```python
from build123d import *

# Parameters (mm, degrees)
SKETCH1_R           = 1.6
SKETCH1_W           = 21
SKETCH1_H           = 41
BOSS_EXTRUDE1_DEPTH = 11
SKETCH6_W           = 21
SKETCH6_H           = 0.1
CUT_EXTRUDE1_DEPTH  = 91.428148273
SKETCH7_W           = 21
SKETCH7_H           = 41.2
SKETCH7_R           = 1.6
CUT_EXTRUDE2_DEPTH  = 11
BOSS_EXTRUDE2_START = -11
SKETCH8_W           = 200
SKETCH8_H           = 250
SKETCH8_W_2         = 21
SKETCH8_H_2         = 41.2
SKETCH8_R           = 1.6
BOSS_EXTRUDE2_DEPTH = 11
FILLET1_R           = 64
FILLET2_R           = 64
FILLET3_R           = 64
FILLET4_R           = 64
SKETCH12_R          = 6.933523759
BOSS_EXTRUDE3_DEPTH = 19.05
SKETCH13_R          = 15
CUT_EXTRUDE3_DEPTH  = 11


with BuildPart() as part:
    # Sketch1 → Boss-Extrude1 (new body)
    with BuildSketch(Plane.XY):
        with BuildLine():
            Line((-20, 70), (-20, -50))
            ThreePointArc((-20, -50), (-2.5, -67.5), (15, -50))
            Line((15, -50), (15, 70))
            ThreePointArc((15, 70), (-2.5, 87.5), (-20, 70))
        make_face()
        with Locations((-7.5, 79.5)):
            Circle(SKETCH1_R, mode=Mode.SUBTRACT)
        with Locations(Location((2.5, 79.5, 0), (0, 0, 180))):
            Circle(SKETCH1_R, mode=Mode.SUBTRACT)
        with Locations((2.5, 30.5)):
            Circle(SKETCH1_R, mode=Mode.SUBTRACT)
        with Locations(Location((-7.5, 30.5, 0), (0, 0, 180))):
            Circle(SKETCH1_R, mode=Mode.SUBTRACT)
        with Locations((-2.5, 55)):
            Rectangle(SKETCH1_W, SKETCH1_H, mode=Mode.SUBTRACT)
    extrude(amount=BOSS_EXTRUDE1_DEPTH)

    # Sketch6 → Cut-Extrude1 (cut, through all)
    with BuildSketch(Plane.XY.offset(11)):
        with Locations((-2.5, 75.55)):
            Rectangle(SKETCH6_W, SKETCH6_H)
        with Locations((-2.5, 34.45)):
            Rectangle(SKETCH6_W, SKETCH6_H)
    extrude(amount=-CUT_EXTRUDE1_DEPTH, mode=Mode.SUBTRACT)

    # Sketch7 → Cut-Extrude2 (cut)
    with BuildSketch(Plane(origin=(0, 0, 0), x_dir=(-1, 0, 0), z_dir=(0, 0, -1))):
        with Locations((2.5, -35)):
            Rectangle(SKETCH7_W, SKETCH7_H)
        with Locations((-2.5, -10.5)):
            Circle(SKETCH7_R)
        with Locations((7.5, -10.5)):
            Circle(SKETCH7_R)
        with Locations((-2.5, -59.5)):
            Circle(SKETCH7_R)
        with Locations((7.5, -59.5)):
            Circle(SKETCH7_R)
    extrude(amount=-CUT_EXTRUDE2_DEPTH, mode=Mode.SUBTRACT)

    # Sketch8 → Boss-Extrude2 (add)
    # profile 1 of 6: a face of its own
    with BuildSketch(Plane.XY.offset(11).offset(BOSS_EXTRUDE2_START)):
        with Locations((-2.5, 55)):
            Rectangle(SKETCH8_W, SKETCH8_H)
        with BuildLine():
            ThreePointArc((-20, -50), (-2.5, -67.5), (15, -50))
            Line((15, -50), (15, 70))
            ThreePointArc((15, 70), (-2.5, 87.5), (-20, 70))
            Line((-20, 70), (-20, -50))
        make_face(mode=Mode.SUBTRACT)
    # profile 2 of 6: a face of its own
    with BuildSketch(Plane.XY.offset(11).offset(BOSS_EXTRUDE2_START)):
        with Locations((-2.5, -35)):
            Rectangle(SKETCH8_W_2, SKETCH8_H_2)
    # profile 3 of 6: a face of its own
    with BuildSketch(Plane.XY.offset(11).offset(BOSS_EXTRUDE2_START)):
        with Locations((-7.5, -59.5)):
            Circle(SKETCH8_R)
    # profile 4 of 6: a face of its own
    with BuildSketch(Plane.XY.offset(11).offset(BOSS_EXTRUDE2_START)):
        with Locations((2.5, -59.5)):
            Circle(SKETCH8_R)
    # profile 5 of 6: a face of its own
    with BuildSketch(Plane.XY.offset(11).offset(BOSS_EXTRUDE2_START)):
        with Locations((-7.5, -10.5)):
            Circle(SKETCH8_R)
    # profile 6 of 6: a face of its own
    with BuildSketch(Plane.XY.offset(11).offset(BOSS_EXTRUDE2_START)):
        with Locations((2.5, -10.5)):
            Circle(SKETCH8_R)
    extrude(amount=BOSS_EXTRUDE2_DEPTH)

    # Fillet1
    fillet1_edges = [part.edges().sort_by_distance(p)[0] for p in [
        (-102.5, 180, 5.5),
    ]]
    fillet(fillet1_edges, radius=FILLET1_R)

    # Fillet2
    fillet2_edges = [part.edges().sort_by_distance(p)[0] for p in [
        (97.5, 180, 5.5),
    ]]
    fillet(fillet2_edges, radius=FILLET2_R)

    # Fillet3
    fillet3_edges = [part.edges().sort_by_distance(p)[0] for p in [
        (97.5, -70, 5.5),
    ]]
    fillet(fillet3_edges, radius=FILLET3_R)

    # Fillet4
    fillet4_edges = [part.edges().sort_by_distance(p)[0] for p in [
        (-102.5, -70, 5.5),
    ]]
    fillet(fillet4_edges, radius=FILLET4_R)

    # Sketch12 → Boss-Extrude3 (add)
    with BuildSketch(Plane(origin=(0, 0, 0), x_dir=(-1, 0, 0), z_dir=(0, 0, -1))):
        with Locations(Location((67.5, 155, 0), (0, 0, 180))):
            Circle(SKETCH12_R)
        with Locations(Location((-62.5, -45, 0), (0, 0, 180))):
            Circle(SKETCH12_R)
        with Locations(Location((67.5, -45, 0), (0, 0, 180))):
            Circle(SKETCH12_R)
        with Locations(Location((-62.5, 155, 0), (0, 0, 180))):
            Circle(SKETCH12_R)
    extrude(amount=BOSS_EXTRUDE3_DEPTH)

    # Sketch13 → Cut-Extrude3 (cut)
    with BuildSketch(Plane.XY.offset(11)):
        with Locations((-62.5, 135)):
            Circle(SKETCH13_R)
        with Locations((57.5, 135)):
            Circle(SKETCH13_R)
        with Locations((57.5, -25)):
            Circle(SKETCH13_R)
        with Locations((-62.5, -25)):
            Circle(SKETCH13_R)
    extrude(amount=-CUT_EXTRUDE3_DEPTH, mode=Mode.SUBTRACT)


solid = part.part
```
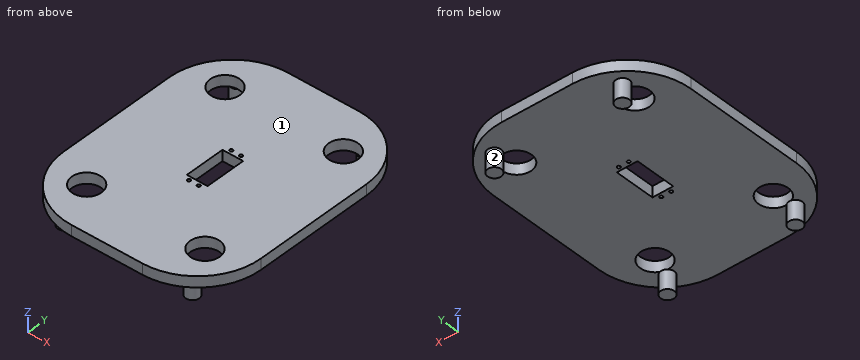
Part model, mm, in its own coordinate system. Face numbers are marked on the shaded views. Coordinates: 2 decimals unless noted, no trailing zeros. Order: outer loops, then holes, each group sorted by start corner. A loop starts at its lowest first (then second) coordinate and runs counter-clockwise, first axis right, second up. Notation, with made-up numbers: (-20, 77.5) - (10, 77.5) arc R8 cw to (10, 89.5) - close; hole circle Ø9 at (71.25, -10). An arc over 180 degrees is marked (long way). Return JSON: item names as keys, results as strings. Group by question number.
Item 1: Cut at B-B (z = -4). List the corners of the cut face in (x, y), plus the area to 3 significant figures.
Item 2: Cut at D-D (x = 19.5). List the corners of the cut face in (y, z).
Item 3: Pull direction X, two halves, no side cores. Call the marked faces 1 and 2: pulls with the +X half, pulls with the -X half, needs draft (parallel to the pull), parting line crosses it, or undercut.
Item 4: Cut at A-A (y = -15). List the corners of the cut face in (x, z), plus the area to 3 significant figures.
Item 5: Cut at C-C (y = 155). List the corners of the cut face in (x, z), plus the area to 3 significant figures.
Item 6: Pin check, flat tips, straight feed: pin 1 (4 mm diameter, centred on x = -7.5, y = 30.5, fed in from -Z); pin 2 (2 mm diameter, centred on x = -64.5, y = -38.5, fed in from +Z); pin 3 (5 mm diameter, centred on y = 153, z = 3.5, fed in from -X) (3 decimals). Stop position of each tip, or through.
Item 7: Drill centre lines: probe 1 along Y at (x, z) = (-7.5, 6.25); probe 2 along Y at (x, z) = (-5, 0.5); probe 3 along Y at (x, z) = (57, 7). Where is each one in solid material? Low to high. Write a range as from..to.
Check values:
{
 "1": {"outline": "circle Ø13.87 at (-67.5, -45); circle Ø13.87 at (-67.5, 155); circle Ø13.87 at (62.5, -45); circle Ø13.87 at (62.5, 155)", "area": "604 mm2"},
 "2": {"outline": "(-70, 0) - (180, 0) - (180, 11) - (-70, 11) - close"},
 "3": {"face 1": "needs draft", "face 2": "undercut"},
 "4": {"outline": "(-101.86, 0) - (-73.68, 0) - (-73.68, 11) - (-101.86, 11) - close; (-51.32, 0) - (46.32, 0) - (46.32, 11) - (-51.32, 11) - close; (68.68, 0) - (96.86, 0) - (96.86, 11) - (68.68, 11) - close", "area": "1,690 mm2"},
 "5": {"outline": "(-89.24, 0) - (-74.43, 0) - (-74.43, -19.05) - (-60.57, -19.05) - (-60.57, 0) - (55.57, 0) - (55.57, -19.05) - (69.43, -19.05) - (69.43, 0) - (84.24, 0) - (84.24, 11) - (-89.24, 11) - close", "area": "2,440 mm2"},
 "6": {"pin 1": "stops at z = 0", "pin 2": "stops at z = 0", "pin 3": "stops at x = -92.405"},
 "7": {"probe 1": "y = -70..28.9, 32.1..34.4, 75.6..77.9, 81.1..180", "probe 2": "y = -70..34.4, 75.6..180", "probe 3": "y = -65.53..-39.99, -10.01..120.01, 149.99..175.53"}
}
